Geometry check sheet. Reference: the model listing, model coordinates, mm. A direction names the side the tool comes from. Give positions to 0.01 mm unless a question says otherwise; leave off trailing zeros. Write each loop counter-clockwise with the first axis right and the second up, starting at its lowest first coordinate (ties: lowest second). Pieces come first, ordered by that corner, then holes.
(1) Cross-section at C-C (z = 5.75). Record the boundary of the cut face in (x, y).
(2) Cross-section at D-D (x = 141.5). Record the boundary of the cut face in (y, z), and give its area (3 significant figures).
(3) Cross-section at B-B (y = -12.5). Record the boundary of the cut face in (x, z).
(4) Cross-section at A-A (x = 75.5). Record the boundary of the cut face in (y, z), and give its area (3 significant figures).
(5) Depth check by flat-ended pin: P1, Ø1.5, axis at x = 132, z = 2.5, coming from the +Y side; P2, Ø6.5, axis at x = 44, y = -9, coming from the -Z side; P3, Ø6, axis at y = -12, z = 10, coming from the -X side; P4, Ø6.5, axis at x = 106.5, z = 6.5, coming from the +Y side. Enter the tip coordinate at first touch or a pass-through.
(6) Thickness scan on line 1 along Z through (x, y) = (21, -1.75); line 2 along Y through (x, z) = (91, -0.5); line 3 along X through (y, z) = (-16.5, 9.25). Record the ranges inside material, lowest first.
(7) Tool access check on faces 1 (the flat face through (78, 6.35, 15)), 2 (the flat face through (78, -5, 13.874)). Record the directions out of +Z, -Z, +X, -X, +Y, -Y that give a thin tool (end or side, any length) a straight path to the whole face; none if there is none.
```python
from build123d import *

# Parameters (mm, degrees)
SALIENTE_EXTRUIR1_DEPTH = 158
CORTAR_EXTRUIR3_DEPTH   = 105
CORTAR_EXTRUIR4_DEPTH   = 105


with BuildPart() as part:
    # Croquis1 → Saliente-Extruir1 (new body)
    with BuildSketch(Plane(origin=(0, 0, 0), x_dir=(0, 0, -1), z_dir=(1, 0, 0))):
        Polygon((-16.874298957, 6.35), (-16.874298957, -19.05), (8.525701043, -19.05), (8.525701043, -16.05), (-13.874298957, -16.05), (-13.874298957, 6.35), align=None)
    extrude(amount=SALIENTE_EXTRUIR1_DEPTH)

    # Croquis3 → Cortar-Extruir3 (cut)
    with BuildSketch(Plane(origin=(0, 6.35, 0), x_dir=(1, 0, 0), z_dir=(0, 1, 0))):
        Polygon((0, -16.874298957), (25.4, 8.525701043), (0, 8.525701043), align=None)
    extrude(amount=-CORTAR_EXTRUIR3_DEPTH, mode=Mode.SUBTRACT)

    # Croquis4 → Cortar-Extruir4 (cut)
    with BuildSketch(Plane(origin=(0, 6.35, 0), x_dir=(1, 0, 0), z_dir=(0, 1, 0))):
        Polygon((158, -16.874298957), (158, 8.525701043), (132.6, 8.525701043), align=None)
    extrude(amount=-CORTAR_EXTRUIR4_DEPTH, mode=Mode.SUBTRACT)


solid = part.part
```
Reply:
1. outline: (11.12, -19.05) - (146.88, -19.05) - (146.88, -16.05) - (11.12, -16.05) - close
2. outline: (-19.05, 0.37) - (-16.05, 0.37) - (-16.05, 13.87) - (6.35, 13.87) - (6.35, 16.87) - (-19.05, 16.87) - close
2. area: 117 mm2
3. outline: (0, 16.87) - (3, 13.87) - (155, 13.87) - (158, 16.87) - close
4. outline: (-19.05, -8.53) - (-16.05, -8.53) - (-16.05, 13.87) - (6.35, 13.87) - (6.35, 16.87) - (-19.05, 16.87) - close
4. area: 143 mm2
5. P1: stops at y = -16.05
5. P2: stops at z = 13.87
5. P3: passes through
5. P4: stops at y = -16.05
6. line 1: z = 13.87 to 16.87
6. line 2: y = -19.05 to -16.05
6. line 3: x = 7.62 to 150.38
7. face 1: +Z, -Z, +X, -X, +Y
7. face 2: -Z, +X, -X, +Y
